Design review of the part built by this model. Coordinates are the model's own, in mm. Face numbers are marked on the shaded views. A direction names the side the tool comes from. Coordinates: 2 decimals unless noted, no trailing zeros. Loops run counter-clockwise (first coordinate to the right, second up) from the corner with the lowest first, then second, coordinate; pieces in that order, holes last. Notation, with made-up numbers: M 55,8 L 112,8 A11 cw 112,12 Z; hole C 25,15.5 d8. An arc over 180 degrees is marked long. Put each result on its own line as item: value. Start each with the question number.
(1) Take a section at C-C, the plane z = 10. Give the boundary of the cut face in (x, y), then the cut area to 3 significant figures.
(2) For probe 1 along Z at (x, y) = (8.5, 121); probe 2 along Y at (x, z) = (-4, -7); probe 3 along Y at (x, z) = (1, -5), list the stretches that pass through material, from the lowest coordinate up. Write a range as [from, to].
(3) Take a section at B-B, the plane y = 133. Give the boundary of the cut face in (x, z), then the cut area to 3 significant figures.
(4) For the marked faces 1 and 2, list the 3-axis set-ups (+Z, -Z, +X, -X, +Y, -Y) from which the entire face can be reached by the end or side of a thin tool; tool diameter is ignored.
(5) Take a section at A-A, the plane x = 1. Give the boundary of the cut face in (y, z), then the cut area to 3 significant figures.
(6) Take a section at D-D, the plane x = -5. Give the boundary of the cut face in (y, z).
(7) Clearance check with flat-ended pins moving along their axes: pin 1 (2 mm diameter, centred on x = 3, z = -10, fed in from +Y); pin 2 (8 mm diameter, centred on x = -7.5, y = 137.5, fed in from +Z); pin 3 (4 mm diameter, centred on x = -4.5, z = 17.5, fed in from +Y). State where each tip first meets the part, or that it passes through.
```python
from build123d import *

# Parameters (mm, degrees)
BOSS_EXTRUDE1_DEPTH = 22.5
CUT_EXTRUDE1_DEPTH  = 36


with BuildPart() as part:
    # Sketch1 → Boss-Extrude1 (new body, symmetric)
    with BuildSketch(Plane.XY):
        with BuildLine():
            Line((-17.5, 148.975669154), (-17.5, 30.31))
            Line((-17.5, 30.31), (17.5, 30.31))
            Line((17.5, 30.31), (17.5, 148.975669154))
            ThreePointArc((17.5, 148.975669154), (0, 150), (-17.5, 148.975669154))
        make_face()
    extrude(amount=BOSS_EXTRUDE1_DEPTH, both=True)

    # Sketch2 → Cut-Extrude1 (cut, through all)
    with BuildSketch(Plane(origin=(17.5, 0, 0), x_dir=(0, 0, -1), z_dir=(1, 0, 0))):
        Polygon((-22.5, 84.019237886), (-7.5, 110), (-7.5, 150), (-22.5, 150), align=None)
    extrude(amount=-CUT_EXTRUDE1_DEPTH, mode=Mode.SUBTRACT)


solid = part.part
```
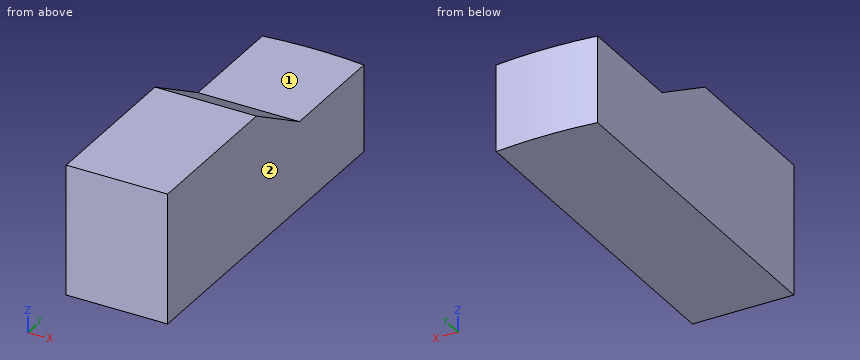
Computed values:
1. outline: M -17.5,30.31 L 17.5,30.31 L 17.5,105.67 L -17.5,105.67 Z
1. area: 2,640 mm^2
2. probe 1: z = [-22.5, 7.5]
2. probe 2: y = [30.31, 149.95]
2. probe 3: y = [30.31, 150]
3. outline: M -17.5,-22.5 L 17.5,-22.5 L 17.5,7.5 L -17.5,7.5 Z
3. area: 1,050 mm^2
4. face 1: +Z, +X, -X, +Y
4. face 2: +Z, -Z, +X, +Y, -Y
5. outline: M 30.31,-22.5 L 150,-22.5 L 150,7.5 L 110,7.5 L 84.02,22.5 L 30.31,22.5 Z
5. area: 4,590 mm^2
6. outline: M 30.31,-22.5 L 149.92,-22.5 L 149.92,7.5 L 110,7.5 L 84.02,22.5 L 30.31,22.5 Z
7. pin 1: stops at y = 149.99
7. pin 2: stops at z = 7.5
7. pin 3: stops at y = 96.14
